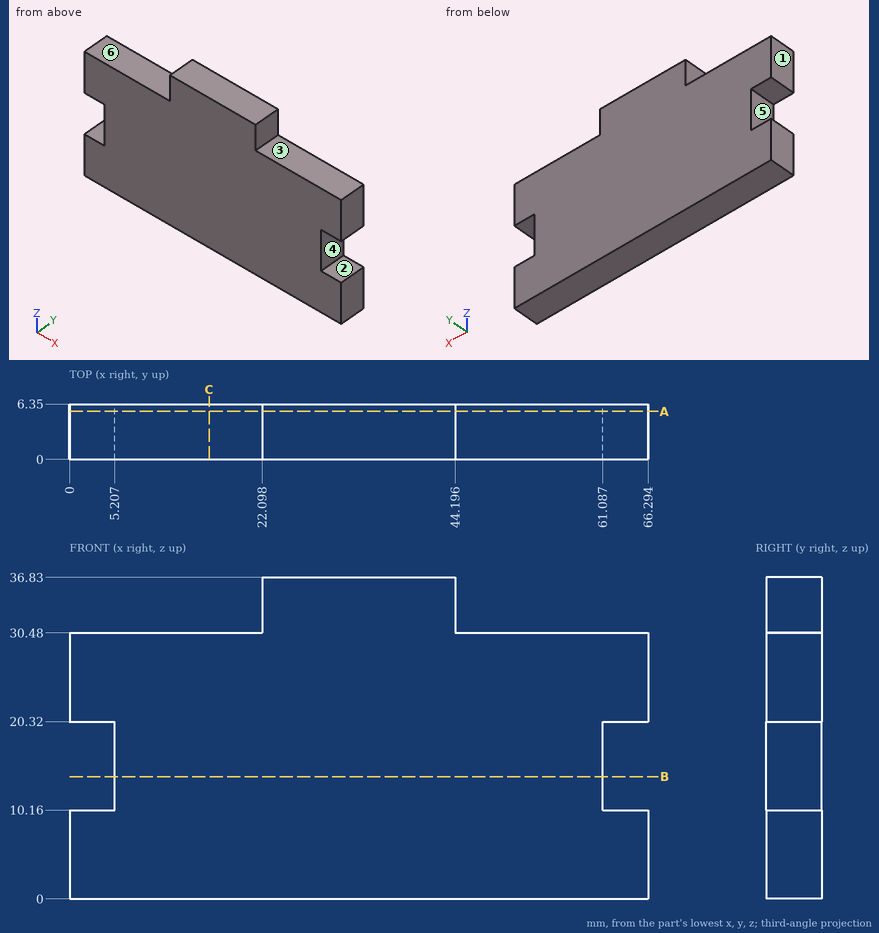
Input: dimensioned drawing with shaded views. Units: mm. Origin: part minimum x, y, z. A direction names the side the tool comes from. Give positions to 0.01 mm unless a question says otherwise; leave off trailing zeros. Write each loop counter-clockwise with the first axis right and the second up, starting at its lowest first coordinate (ties: lowest second). Pieces come first, ordered by that corner, then holes.
Q1. Pull-direction query (Z, two-part tool) for the marked faces 1, 2 and 3; classes: pulls with the +Z half, pulls with the -Z half, needs draft (parallel to the pull), parting line crosses it, or undercut.
Q2. Section C-C, the plane x = 16. Output: boundary loops of the cut face in (y, z), plus the area to 3 significant figures.
Q3. Section B-B, the plane z = 14. Output: boundary loops of the cut face in (x, y).
Q4. First-contact query: P1, Ø3, axis at y = 2.5, z = 15, coming from the -X side; P2, Ø1.9, axis at x = 51.5, y = 4.5, coming from the +Z side; P3, Ø3, axis at y = 2.5, z = 35, coming from the -X side. Flat tips, straight axial feed; report the tip coordinate or a pass-through.
Q5. Section A-A, the plane y = 5.5. Output: boundary loops of the cut face in (x, z), plus the area to 3 significant figures.
Q6. Material intervals for probe 1 along Z at (x, y) = (3.5, 3.75); probe 2 along X at (y, z) = (4.5, 15.5); probe 3 along Z at (x, y) = (58, 1), sorted ascending.
Q7. Set-up query: the marked faces 4, 5 and 6. Return all of +Z, -Z, +X, -X, +Y, -Y with unobstructed straight access to the full face (end or side cutting, diameter ignored); none if empty.
Filled in:
1. face 1: needs draft
1. face 2: undercut
1. face 3: pulls with the +Z half
2. outline: (0, 0) - (6.35, 0) - (6.35, 30.48) - (0, 30.48) - close
2. area: 194 mm2
3. outline: (5.21, 0) - (61.09, 0) - (61.09, 6.35) - (5.21, 6.35) - close
4. P1: stops at x = 5.21
4. P2: stops at z = 30.48
4. P3: stops at x = 22.1
5. outline: (0, 0) - (66.29, 0) - (66.29, 10.16) - (61.09, 10.16) - (61.09, 20.32) - (66.29, 20.32) - (66.29, 30.48) - (44.2, 30.48) - (44.2, 36.83) - (22.1, 36.83) - (22.1, 30.48) - (0, 30.48) - (0, 20.32) - (5.21, 20.32) - (5.21, 10.16) - (0, 10.16) - close
5. area: 2,060 mm2
6. probe 1: z = 0 to 10.16, 20.32 to 30.48
6. probe 2: x = 5.21 to 61.09
6. probe 3: z = 0 to 30.48
7. face 4: +X, +Y, -Y
7. face 5: -X, +Y, -Y
7. face 6: +Z, -X, +Y, -Y
